The listing builds one solid part. Answer for the finished solid, in the listing's coordinates (mm). Face numbers are marked on the shaded views. A direction names the side the tool comes from. Give positions to 0.01 mm unless a question says otherwise; leave off trailing zeros. Order: outer loops, then holes, each group sorted by start corner. A loop starts at its lowest first (then second) coordinate and runs counter-clockwise, first axis right, second up.
Solid Edge part; units mm, degrees
sketch "Sketch1" plane through (0, 0, 0) normal (0, 0, 1) x (1, 0, 0)
  line L0 (4, 0) -> (4, 20)
  line L1 (0, 20) -> (4, 20)
  line L2 (0, 0) -> (0, 20)
  line L3 (0, 0) -> (0, -8)
  line L4 (0, -8) -> (6.5, -8)
  line L5 (6.5, -8) -> (6.5, 0)
  line L6 (6.5, 0) -> (4, 0)
revolve "RevolvedProtrusion1" add sketch "Sketch1" angle 360 about axis through (0, 0, 0) along (0, 1, 0)
sketch "Sketch2" plane through (0, 0, 0) normal (1, 0, 0) x (0, 1, 0)
  line L0 (-8, 3.8415) -> (-4, 3.8415)
  line L1 (-1.7821, 0) -> (-4, 3.8415)
  line L2 (-8, 0) -> (-1.7821, 0)
  line L3 (-8, 0) -> (-8, 3.8415)
revolve "RevolvedCutout1" cut sketch "Sketch2" angle 360 about axis through (0, -4.5, 0) along (0, 1, 0)
sketch "Sketch3" plane through (0, -8, 0) normal (0, -1, 0) x (0, 0, 1)
  circle A0 centre (0, 0) radius 3.8415
  line L0 (-3, -1.7321) -> (0, -3.4641)
  line L1 (0, -3.4641) -> (3, -1.7321)
  line L2 (3, -1.7321) -> (3, 1.7321)
  line L3 (3, 1.7321) -> (0, 3.4641)
  line L4 (0, 3.4641) -> (-3, 1.7321)
  line L5 (-3, 1.7321) -> (-3, -1.7321)
extrude "Protrusion1" add sketch "Sketch3" against normal up to next
sketch "Sketch4" plane through (0, 0, 0) normal (0, 0, 1) x (1, 0, 0)
  line L0 (-3.4641, -8) -> (0, -8)
  line L1 (0, -8) -> (0, -7.0718)
  line L2 (0, -7.0718) -> (-3.4641, -8)
revolve "RevolvedCutout2" cut sketch "Sketch4" angle 360 about axis through (0, -4.5, 0) along (0, 1, 0)
fillet "Round1" radius 0.4 1 edges at (0, 0, -4)
fillet "Round2" radius 0.65 1 edges at (0, -8, -6.5)
chamfer "倒斜角_2" distance 0.5333 angle 45 1 edges at (0, 20, -4)
cosmetic_thread "螺纹_3" thread depth 16
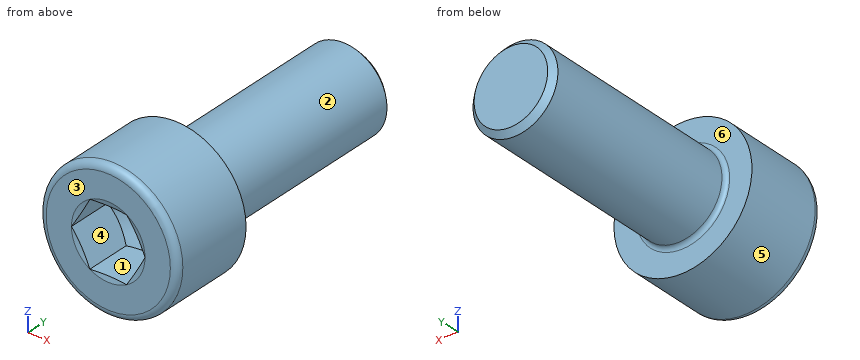
1) Given P1, Ø2, axis at x = -3.5, y = 11, coming from the +Z side; P2, Ø1.5, axis at x = -4, y = -1.5, coming from the +Z side; P3, Ø6, axis at y = 17, z = 1.5, coming from the +X side, each flat-ended and moving along its own axis, determine where each tip first touches the part or whether it passes through.
Geometry says:
P1: stops at z = 3.12
P2: stops at z = 5.63
P3: stops at x = 4
2) A tool of negligible diameter and unlimited length cuts with its end or side. For the marked faces 4, 5 and 6, from which of +Z, -Z, +X, -X, +Y, -Y can it reach the whole face along a straight path? Write none if from no direction.
Geometry says:
face 4: -Y
face 5: +Y, -Y
face 6: +Y
3) For a pull along Z with two mould halves and no side action, classify the marked faces 1, 2 and 3 as +Z half, -Z half, draft (parallel to the pull), parting line (faces both ways), or undercut.
Geometry says:
face 1: undercut
face 2: parting line
face 3: draft
4) Find section A-A (y = 9.75). Write down the section's boundary in (x, z), then the cut area to 3 significant figures.
Geometry says:
outline: circle Ø8 at (0, 0)
area: 50.3 mm2
5) Straight lines are drawn through the part: probe 1 along Y at (x, z) = (2, 5); probe 2 along X at (y, z) = (19.25, 2); probe 3 along Z at (x, y) = (-2.25, -4). For each, find the intervals that lie inside material, in ascending order.
Geometry says:
probe 1: y = -8 to 0
probe 2: x = -3.46 to 3.46
probe 3: z = -6.1 to -2.1, 2.1 to 6.1
